Could you check a few things on this drawing? It's one solid part, dimensions in mm from its lowest x, y, z. A direction names the side the tool comes from. Give positions to 0.01 mm unless a question says otherwise; leave off trailing zeros. Loops run counter-clockwise (first coordinate to the right, second up) from the corner with the lowest first, then second, coordinate; pieces in that order, holes last. Notation, with made-up numbers: (44.5, 64) -> (72.5, 64) arc R20 cw to (72.5, 78) -> close; hole circle Ø6 at (37.5, 63). An arc over 180 degrees is marked (long way). One line per question, with ' | ' between items.
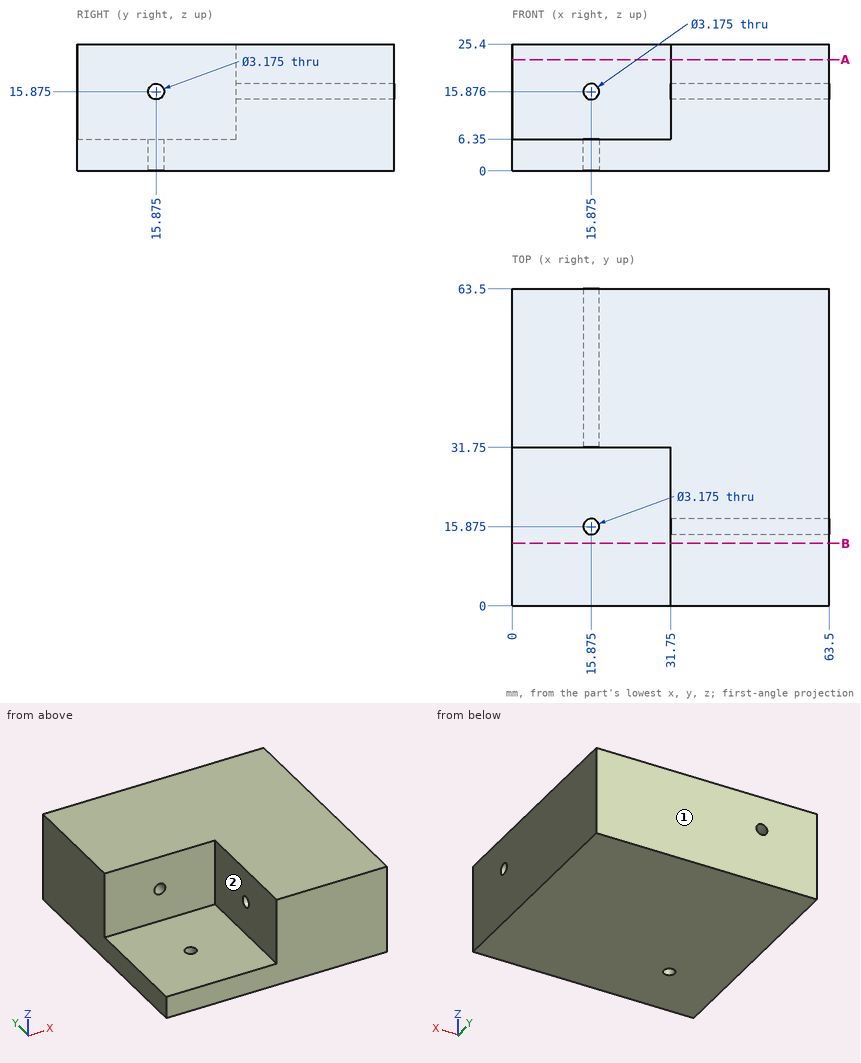
Q1. If we section it at B-B (y = 12.5): Write out the boundary of the cut face in (x, z), plus the area to 3 significant figures.
Entries:
outline: (0, 0) -> (63.5, 0) -> (63.5, 25.4) -> (31.75, 25.4) -> (31.75, 6.35) -> (0, 6.35) -> close | area: 1,010 mm²
Q2. On a 3-axis mill with a long thin cutter (end or side, diameter ignored), from which of +Z, -Z, +X, -X, +Y, -Y can I reach the whole of each face in a straight line? I mean the marked faces 1 and 2. Say none if no direction works.
Entries:
face 1: +Z, -Z, +X, -X, +Y | face 2: +Z, -X, -Y
Q3. For pin 1 Ø5 at (y, z) = (15.875, 15.875) entering from -X; pin 2 Ø5 at (x, z) = (15.88, 15.88) entering from -Y; pin 3 Ø1.9 at (x, y) = (15.875, 15.875) entering from +Z, each with a flat end and sliding along its axis, tell me the tip position at first contact or that it passes through.
Entries:
pin 1: x = 31.75 | pin 2: y = 31.75 | pin 3: through
Q4. If we section it at A-A (z = 22.25): Write out the boundary of the cut face in (x, y), plus the area to 3 significant figures.
Entries:
outline: (0, 31.75) -> (31.75, 31.75) -> (31.75, 0) -> (63.5, 0) -> (63.5, 63.5) -> (0, 63.5) -> close | area: 3,020 mm²
Q5. If I drill on probe 1 along X at (y, z) = (9.5, 18.5); probe 2 along X at (y, z) = (33.5, 16.5) (1 decimal), over which ranges is the centre line in solid material (lowest first)? Write a range as from..to.
Entries:
probe 1: 31.75..63.5 | probe 2: 0..14.4, 17.3..63.5
